CAD build for the part. Positions are in the model's coordinates, mm. A direction names the side the tool comes from. Round coordinates to 2 decimals unless told otherwise and drop trailing zeros. Loops run counter-clockwise (first coordinate to the right, second up) from the corner with the lowest first, then second, coordinate; pieces in that order, holes last. Notation, with made-up numbers: (-33, 30.25) - (23, 30.25) arc R9 cw to (23, 44.25) - close; hole circle Ø5 at (-7, 14). An arc over 180 degrees is marked (long way). Use one line per item in the form item = value.
from build123d import *

# Parameters (mm, degrees)
SKETCH4_R                      = 4.025
BOSS_EXTRUDE1_DEPTH            = 10
SWEEP2_START                   = -10
SWEEP2_DEPTH                   = 20
CUT_EXTRUDE2_REACH             = 58.724
BOSS_EXTRUDE2_DEPTH            = 20
CUT_EXTRUDE3_REACH             = 69.223
SKETCH4_10_R                   = 4.025
CUT_EXTRUDE3_DIRECTION_2_DEPTH = 68.223447839
FILLET4_R                      = 10
F_6_CLEARANCE_HOLE1_D          = 3.7973


with BuildPart() as part:
    # Sketch4 → Boss-Extrude1 (new body)
    # profile 1 of 2: a face of its own
    with BuildSketch(Plane.XY):
        with BuildLine():
            Line((-10, 10), (25, 10))
            Line((25, 10), (25, -10))
            Line((25, -10), (-10, -10))
            ThreePointArc((-10, -10), (-13.535533906, -8.535533906), (-15, -5))
            Line((-15, -5), (-15, 5))
            ThreePointArc((-15, 5), (-13.535533906, 8.535533906), (-10, 10))
        make_face()
        Circle(SKETCH4_R, mode=Mode.SUBTRACT)
    # profile 2 of 2: a face of its own
    with BuildSketch(Plane.XY):
        Circle(SKETCH4_R)
    extrude(amount=-BOSS_EXTRUDE1_DEPTH)

    # Sweep2: read off the stored shape, not the designer's step
    # Sweep2 outline → Sweep2 (add)
    with BuildSketch(Plane(origin=(0, 0, 0), x_dir=(1, 0, 0), z_dir=(0, 1, 0)).offset(SWEEP2_START)):
        Polygon((40.170370869, -5.058020855), (40.170370869, -18.294095226), (49.829629131, -15.705904774), (49.829629131, 1.058020855), (38.67117676, 6.336819228), (25, 10), (25, 0), (35.32882324, -2.767599846), align=None)
    extrude(amount=SWEEP2_DEPTH)

    # Sketch18 → Cut-Extrude2 (cut, up to next)
    with BuildSketch(Plane(origin=(0, 10, 0), x_dir=(1, 0, 0), z_dir=(0, 1, 0)), mode=Mode.PRIVATE) as cut_extrude2_sk1:
        Polygon((40.170370869, -18.294095226), (45, -17), (40.170370869, -17), align=None)
    cut_extrude2_tool1 = extrude(cut_extrude2_sk1.sketch, amount=-CUT_EXTRUDE2_REACH, mode=Mode.PRIVATE) & part.part
    add(cut_extrude2_tool1.solids().sort_by_distance((41.780247, 10, 17.431365))[0], mode=Mode.SUBTRACT)

    # Sketch18<3> → Boss-Extrude2 (add, through all)
    with BuildSketch(Plane(origin=(0, 10, 0), x_dir=(1, 0, 0), z_dir=(0, 1, 0))):
        Polygon((49.829629131, -17), (49.829629131, -15.705904774), (45, -17), align=None)
    extrude(amount=-BOSS_EXTRUDE2_DEPTH)

    # Mirror1: part across face


with BuildPart() as part_1:
    add(part.part)
    add(part.part.mirror(Plane(origin=(45, 0, 17), x_dir=(1, 0, 0), z_dir=(0, 0, 1))))

    # Sketch4<10> → Cut-Extrude3 (cut, up to next)
    with BuildSketch(Plane.XY, mode=Mode.PRIVATE) as cut_extrude3_sk1:
        with Locations(Location((0, 0, 0), (0, 0, 180))):
            Circle(SKETCH4_10_R)
    cut_extrude3_tool1 = extrude(cut_extrude3_sk1.sketch, amount=-CUT_EXTRUDE3_REACH, mode=Mode.PRIVATE) & part_1.part
    add(cut_extrude3_tool1.solids().sort_by_distance((0, 0, 0))[0], mode=Mode.SUBTRACT)

    # Sketch4<10> → Cut-Extrude3 direction 2 (cut)
    with BuildSketch(Plane.XY):
        with Locations(Location((0, 0, 0), (0, 0, 180))):
            Circle(SKETCH4_10_R)
    extrude(amount=CUT_EXTRUDE3_DIRECTION_2_DEPTH, mode=Mode.SUBTRACT)

    # Fillet4
    # the kernel refuses this fillet: 10 mm, written as the material it adds along each edge
    with BuildSketch(Plane(origin=(25, 10, 34), x_dir=(-1, 0, 0), z_dir=(0, -1, 0))) as fillet4_piece_1:
        with BuildLine():
            CenterArc((FILLET4_R * 0.131652497591, FILLET4_R), FILLET4_R, 255, 15)
            Line((-FILLET4_R * 0.127166547518, FILLET4_R * 0.0340741737128), (0, 0))
            Line((0, 0), (FILLET4_R * 0.131652497591, 0))
        make_face()
    extrude(amount=20)
    with BuildSketch(Plane(origin=(25, 10, 0), x_dir=(-1, 0, 0), z_dir=(0, -1, 0))) as fillet4_piece_2:
        with BuildLine():
            CenterArc((FILLET4_R * 0.131652497591, -FILLET4_R), FILLET4_R, 90, 15)
            Line((-FILLET4_R * 0.127166547518, -FILLET4_R * 0.0340741737128), (0, 0))
            Line((0, 0), (FILLET4_R * 0.131652497591, 0))
        make_face()
    extrude(amount=20)
    with BuildSketch(Plane(origin=(40.170370869, -10, 5.058020855), x_dir=(0, 0, 1), z_dir=(0, 1, 0))) as fillet4_piece_3:
        with BuildLine():
            CenterArc((6.276396903, -10), FILLET4_R, 90, 58.94603144)
            Line((-2.290421009, -4.841547629), (0, 0))
            Line((0, 0), (6.276396903, 0))
        make_face()
    extrude(amount=20)
    with BuildSketch(Plane(origin=(40.170370869, -10, 28.941979145), x_dir=(-0.90395035591234, 0, 0.4276374095492042), z_dir=(0, 1, 0))) as fillet4_piece_4:
        with BuildLine():
            CenterArc((6.355481446, -9.94992531), FILLET4_R, 95.736251166, 58.94603144)
            Line((-2.684022113, -5.673551214), (0, 0))
            Line((0, 0), (5.355988409, 0))
        make_face()
    extrude(amount=20)
    # the kernel refuses this fillet: 10 mm, written as the material it takes off along each edge
    with BuildSketch(Plane(origin=(49.829629131, -25.829480752, -1.058020855), x_dir=(-0.9039503558586357, 0, -0.4276374096627259), z_dir=(0, 1, 0)), Plane(origin=(49.829629131, -25.829480752, 35.058020855), x_dir=(0, 0, -1), z_dir=(0, 1, 0))) as fillet4_2_piece_1:
        with BuildLine():
            CenterArc((FILLET4_R * 0.633179230062, FILLET4_R), FILLET4_R, 205.317717401, 64.682282599)
            Line((-FILLET4_R * 0.270771125796, FILLET4_R * 0.572362590337), (0, 0))
            Line((0, 0), (FILLET4_R * 0.633179230062, 0))
        make_face()
    extrude(amount=51.658961503, mode=Mode.SUBTRACT)
    with BuildSketch(Plane(origin=(38.67117676, -12.257079455, -6.336819228), x_dir=(0.9039503558586354, 0, 0.42763740966272634), z_dir=(0, 1, 0))) as fillet4_2_piece_2:
        with BuildLine():
            CenterArc((FILLET4_R * 0.0902831782122, -FILLET4_R), FILLET4_R, 90, 10.317717402)
            Line((-FILLET4_R * 0.0888232721735, -FILLET4_R * 0.0161702995791), (0, 0))
            Line((0, 0), (FILLET4_R * 0.0902831782122, 0))
        make_face()
    extrude(amount=24.514158911, mode=Mode.SUBTRACT)
    with BuildSketch(Plane(origin=(25, 13.291312439, -10), x_dir=(-1, 0, 0), z_dir=(0, -1, 0)), Plane(origin=(25, 13.291312439, 44), x_dir=(0.9659258262965777, 0, -0.2588190450744948), z_dir=(0, -1, 0))) as fillet4_2_piece_3:
        with BuildLine():
            CenterArc((FILLET4_R * 0.131652497573, -FILLET4_R), FILLET4_R, 90, 14.999999998)
            Line((-FILLET4_R * 0.127166547502, -FILLET4_R * 0.0340741737034), (0, 0))
            Line((0, 0), (FILLET4_R * 0.131652497573, 0))
        make_face()
    extrude(amount=26.582624879, mode=Mode.SUBTRACT)
    with BuildSketch(Plane(origin=(38.67117676, -12.257079455, 40.336819228), x_dir=(0.9039503558586373, 0, -0.42763740966272235), z_dir=(0, 1, 0))) as fillet4_2_piece_4:
        with BuildLine():
            CenterArc((FILLET4_R * 0.0902831782122, FILLET4_R), FILLET4_R, 259.682282598, 10.317717402)
            Line((-FILLET4_R * 0.0888232721735, FILLET4_R * 0.0161702995791), (0, 0))
            Line((0, 0), (FILLET4_R * 0.0902831782122, 0))
        make_face()
    extrude(amount=24.514158911, mode=Mode.SUBTRACT)

    # #6 Clearance Hole1 (through all)
    with Locations(Plane(origin=(49.829629131, 0, 0), x_dir=(0, 0, -1), z_dir=(1, 0, 0))):
        with Locations((-10.773771446, 0), (-23.226228554, 0)):
            Hole(F_6_CLEARANCE_HOLE1_D / 2)


solid = part_1.part
1) Two-plate mould, pull along Z, no slides. Class faces 1 (the flat face through (32.116, -0.14, -8.093)), 2 (the flat face through (32.116, -0.14, 42.093)), 3 (the cylindrical face through (-3.84, -1.21, -4.93)), 4 (the flat face through (4, -2, 34)): +Z half, -Z half, draft (parallel to the pull), parting line (faces both ways), or undercut.
Report:
face_1 = -Z half
face_2 = +Z half
face_3 = draft
face_4 = undercut
2) Slice it at C-C (x = 38.5). Write the cut outline in (y, z).
Report:
outline = (-10, -6.35) - (10, -6.35) - (10, 5.8) - (-10, 5.8) - close; (-10, 28.2) - (10, 28.2) - (10, 40.35) - (-10, 40.35) - close
3) Drill centre lines: probe 1 along Z at (x, y) = (14, 8.5); probe 2 along Z at (x, y) = (45.25, 0); probe 3 along Z at (x, y) = (42.5, 1.5). Where is each one in solid material? Low to high.
Report:
probe_1 = -10 to 0, 34 to 44
probe_2 = -3.13 to 8.88, 12.67 to 21.33, 25.12 to 37.13
probe_3 = -4.53 to 9.61, 11.94 to 22.06, 24.39 to 38.53
4) Slice it at B-B (y = 7.75). Write the cut outline in (x, z), plus the area to 3 significant figures.
Report:
outline = (-14.18, -10) - (23.68, -10) arc R10 ccw to (26.27, -9.66) - (37.8, -6.57) arc R10 ccw to (39.49, -5.95) - (44.11, -3.77) arc R10 ccw to (49.83, 5.27) - (49.83, 28.73) arc R10 ccw to (44.11, 37.77) - (39.49, 39.95) arc R10 ccw to (37.8, 40.57) - (26.27, 43.66) arc R10 ccw to (23.68, 44) - (-14.18, 44) - (-14.18, 34) - (23.68, 34) arc R10 cw to (26.27, 33.66) - (35.33, 31.23) arc R10 cw to (40.17, 22.67) - (40.17, 11.33) arc R10 cw to (35.33, 2.77) - (26.27, 0.34) arc R10 cw to (23.68, 0) - (-14.18, 0) - close
area = 1,480 mm^2
5) Tool access for faces 5 (the cylindrical face through (38.911, -0.14, 6.477)), 6 (the cylindrical face through (-13, -9, 39)): list every direction of +Z, -Z, +X, -X, +Y, -Y with a clear straight run to the whole face (end or side of a thin tool).
Report:
face_5 = -X, +Y, -Y
face_6 = +Z, -Z, -X, -Y
6) Flat gauge pins, fed straight in: pin 1 (9 mm diameter, centred on y = -1.5, z = 14.5, fed in from -X); pin 2 (5 mm diameter, centred on y = 0, z = 23.23, fed in from -X); pin 3 (1.5 mm diameter, centred on x = 41.5, y = 1, fed in from -Z). Where does each tip first touch, or does it go through?
Report:
pin_1 = 40.08
pin_2 = 39.69
pin_3 = -5.35
7) Slice it at D-D (y = 0). State how many separate pieces and enclosed holes the cut face has, plus the area to 3 significant figures.
Report:
separate_pieces = 5
enclosed_holes = 0
area = 1,270 mm^2
8) Slice it at A-A (x = 0). Write the cut outline in (y, z) (3 decimals), plus the area to 3 significant figures.
Report:
outline = (-10, -10) - (-4.025, -10) - (-4.025, 0) - (-10, 0) - close; (-10, 34) - (-4.025, 34) - (-4.025, 44) - (-10, 44) - close; (4.025, -10) - (10, -10) - (10, 0) - (4.025, 0) - close; (4.025, 34) - (10, 34) - (10, 44) - (4.025, 44) - close
area = 239 mm^2
